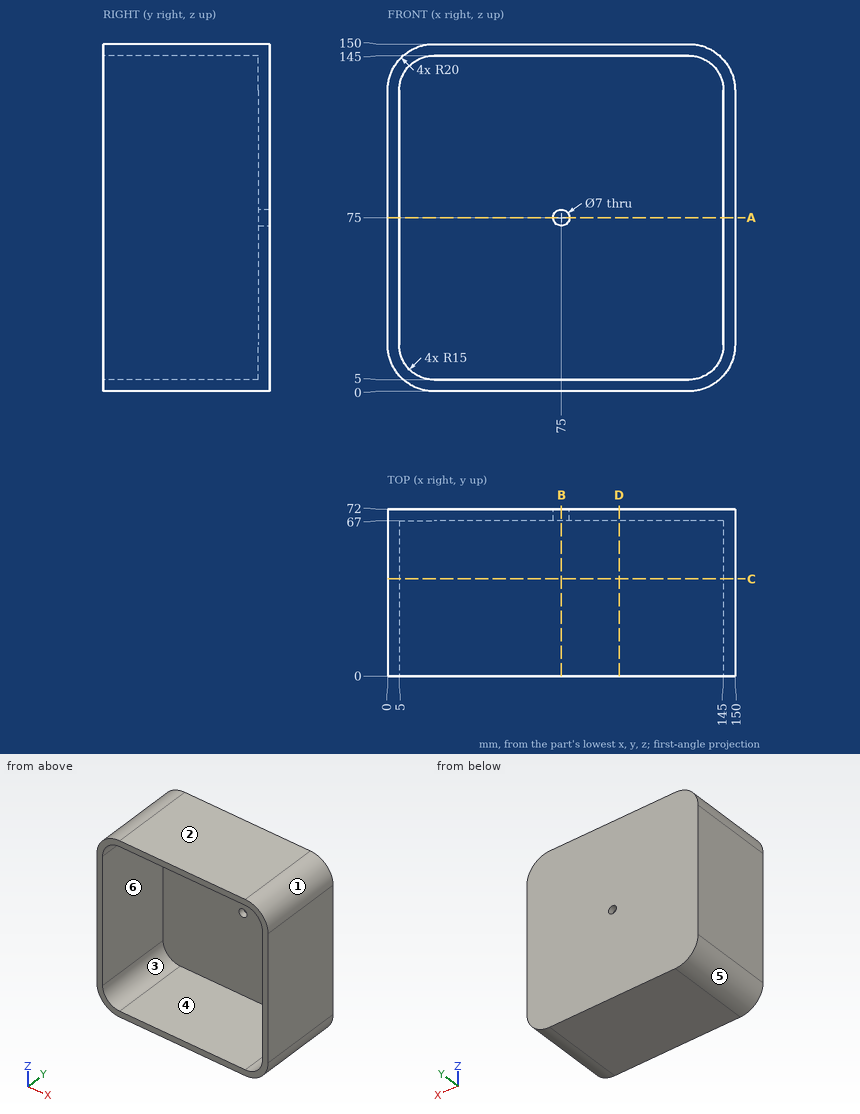
Check sheet for the drawn part. Datum: minimum x, y, z corner. Units: mm. A direction names the side the tool comes from. Give positions to 0.01 mm unless a question says otherwise; leave off trailing zeros. Order: outer loops, then holes, each group sorted by start corner. A loop starts at its lowest first (then second) coordinate and runs counter-clockwise, first axis right, second up. Notation, with made-up numbers: (72, 41.25) - (97, 41.25) arc R26 ccw to (97, 57.25) - close; hole circle Ø7 at (84, 43.25). An arc over 180 degrees is marked (long way). Answer in a Markdown table with one row per item. Add a question column.
Q1. Mould release check, pull along X, two halves, no side actions. Record for the marked faces 1, 2, 3 and 4: pulls with the +X half, pulls with the -X half, needs draft (parallel to the pull), parting line crosses it, or undercut.
Q2. Cross-section at B-B, the plane x = 75. Enter the section's corners in (y, z).
Q3. Tool access check on the marked faces 5 and 6. Record the directions out of +Z, -Z, +X, -X, +Y, -Y that give a thin tool (end or side, any length) a straight path to the whole face; none if there is none.
Q4. Cross-section at C-C, the plane y = 42. Enter the section's corners in (x, z).
Q5. Cross-section at A-A, the plane z = 75. Enter the section's corners in (x, y).
Q6. Material ranges on probe 1 along Z at (x, y) = (47, 59.5); probe 2 along X at (y, z) = (69.6, 75), recorded low to high. Write a range as from..to.
Q7. Gauge pin test, flat end, axial feed: pin 1 (9 mm diameter, centred on x = 75, z = 75, fed in from -Y). Record the tip position at first contact, or that the pin passes through.
Q8. Cross-section at D-D, the plane x = 100. Enter the section's corners in (y, z).
Check values:
| question | item | result |
|---|---|---|
| 1 | face 1 | pulls with the +X half |
| 1 | face 2 | needs draft |
| 1 | face 3 | undercut |
| 1 | face 4 | undercut |
| 2 | outline | (0, 0) - (72, 0) - (72, 71.5) - (67, 71.5) - (67, 5) - (0, 5) - close; (0, 145) - (67, 145) - (67, 78.5) - (72, 78.5) - (72, 150) - (0, 150) - close |
| 3 | face 5 | -Z, -X, +Y, -Y |
| 3 | face 6 | -Y |
| 4 | outline | (0, 20) arc R20 ccw to (20, 0) - (130, 0) arc R20 ccw to (150, 20) - (150, 130) arc R20 ccw to (130, 150) - (20, 150) arc R20 ccw to (0, 130) - close; hole (5, 20) arc R15 ccw to (20, 5) - (130, 5) arc R15 ccw to (145, 20) - (145, 130) arc R15 ccw to (130, 145) - (20, 145) arc R15 ccw to (5, 130) - close |
| 5 | outline | (0, 0) - (5, 0) - (5, 67) - (71.5, 67) - (71.5, 72) - (0, 72) - close; (78.5, 67) - (145, 67) - (145, 0) - (150, 0) - (150, 72) - (78.5, 72) - close |
| 6 | probe 1 | z = 0..5, 145..150 |
| 6 | probe 2 | x = 0..71.5, 78.5..150 |
| 7 | pin 1 | stops at y = 67 |
| 8 | outline | (0, 0) - (72, 0) - (72, 150) - (0, 150) - (0, 145) - (67, 145) - (67, 5) - (0, 5) - close |
